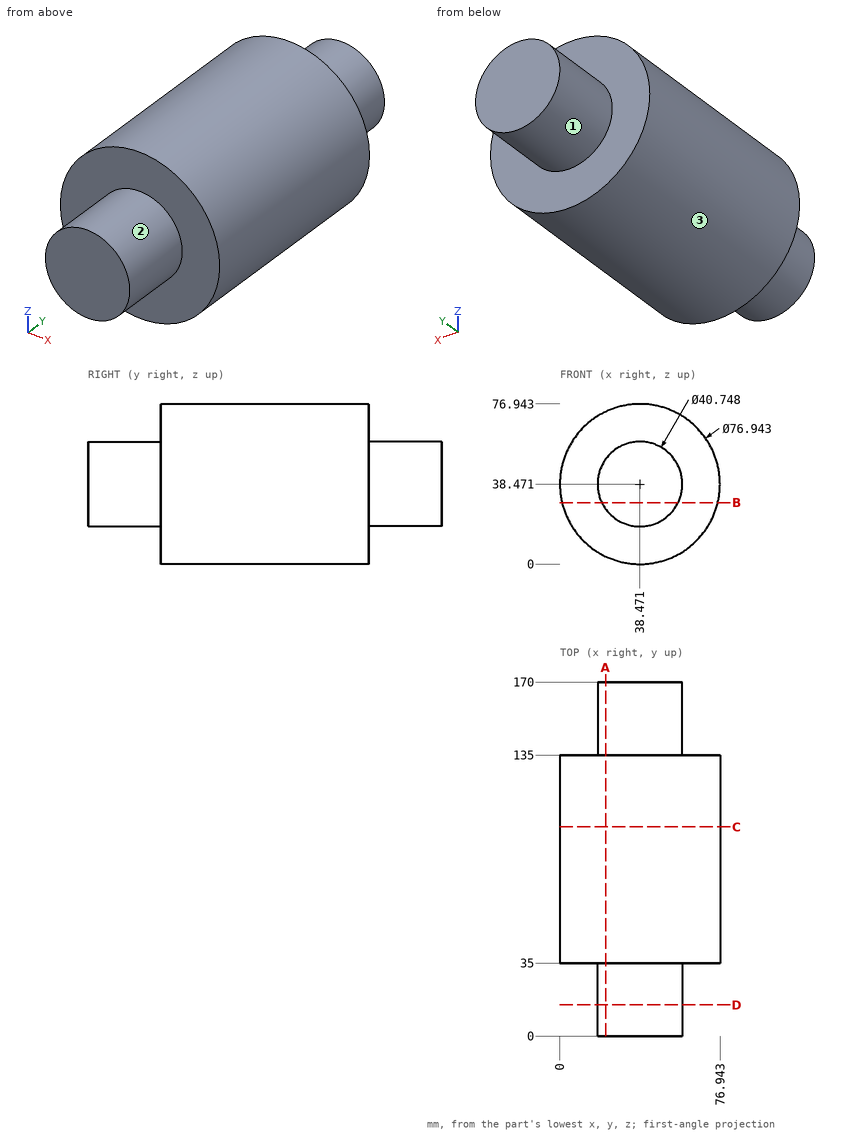
Check sheet for the drawn part. Datum: minimum x, y, z corner. Units: mm. A direction names the side the tool comes from. Round coordinates to 2 decimals unless told otherwise and drop trailing zeros. Order: outer loops, then holes, each group sorted by start corner. A loop starts at its lowest first (then second) coordinate and runs counter-clockwise, first axis right, second up.
(1) Scan lines: probe 1 along Y at (x, z) = (27, 7); probe 2 along Z at (x, y) = (39.5, 33); probe 3 along Z at (x, y) = (37.5, 85). Record each from-to range of solid material in increasing order.
(2) Cross-section at C-C, the plane y = 100.5. Enter the section's corners in (x, z).
(3) Cross-section at B-B, the plane z = 29.5. Enter the section's corners in (x, y), and give its area (3 significant figures).
(4) Cross-section at D-D, the plane y = 15. Enter the section's corners in (x, z) (1 decimal).
(5) Cross-section at A-A, the plane x = 22. Enter the section's corners in (y, z) (1 decimal), and give its area (3 significant figures).
(6) Access from +Z, -Z, +X, -X, +Y, -Y to the whole of each face (thin tool, end or side, straight path). Record for the marked faces 1, 2 and 3.
(7) Go/stop test with flat-tipped pins: P1, Ø8, axis at x = 62.5, z = 8, coming from the -Y side; P2, Ø1, axis at y = 128, z = 27, coming from the -X side; P3, Ø2, axis at x = 32.5, y = 105.5, coming from the +Z side. Record where each tip stops, or that it passes through.
Check sheet entries:
1. probe 1: y = 35 to 135
1. probe 2: z = 18.12 to 58.82
1. probe 3: z = 0.01 to 76.93
2. outline: circle Ø76.94 at (38.47, 38.47)
3. outline: (1.06, 35) - (20.18, 35) - (20.18, 0) - (56.76, 0) - (56.76, 35) - (75.88, 35) - (75.88, 135) - (56.76, 135) - (56.76, 170) - (20.18, 170) - (20.18, 135) - (1.06, 135) - close
3. area: 10,000 mm2
4. outline: circle Ø40.7 at (38.5, 38.5)
5. outline: (0, 26.5) - (35, 26.5) - (35, 3.7) - (135, 3.7) - (135, 26.5) - (170, 26.5) - (170, 50.5) - (135, 50.5) - (135, 73.2) - (35, 73.2) - (35, 50.5) - (0, 50.5) - close
5. area: 8,630 mm2
6. face 1: +Y
6. face 2: -Y
6. face 3: +Y, -Y
7. P1: stops at y = 35
7. P2: stops at x = 1.6
7. P3: stops at z = 76.62
